Read the model definition and answer for the solid it produces. Units are mm, in the model's axes. Face numbers are marked on the shaded views. A direction names the side the tool comes from. Round coordinates to 2 decimals unless told otherwise and drop trailing zeros. Loops run counter-clockwise (first coordinate to the right, second up) from the corner with the lowest first, then second, coordinate; pieces in that order, holes last. Notation, with made-up numbers: (46.5, -13) - (59.5, -13) arc R17 ccw to (59.5, 9) - close; hole circle Ø5 at (55, 53). An arc over 180 degrees is marked (long way). Answer as CSV lines item,"result".
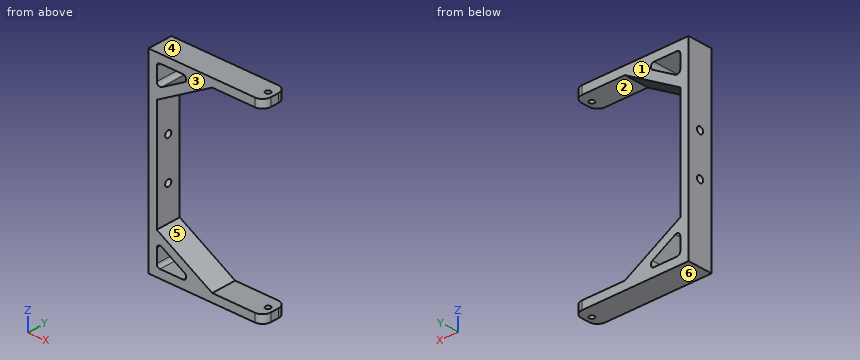
```python
from build123d import *

# Parameters (mm, degrees)
BOSS_EXTRUDE1_DEPTH     = 15
SKETCH2_R               = 1.55
CUT_EXTRUDE1_DEPTH      = 1
CUT_EXTRUDE1_DEPTH_BACK = 116
FILLET1_R               = 2
FILLET2_R               = 5
SKETCH3_R               = 2
CUT_EXTRUDE2_DEPTH      = 6


with BuildPart() as part:
    # Sketch1 → Boss-Extrude1 (new body)
    with BuildSketch(Plane(origin=(0, 0, 0), x_dir=(1, 0, 0), z_dir=(0, 1, 0))):
        Polygon((61.707917854, 52.5), (66.707917854, 52.5), (66.707917854, 57.5), (62.241203502, 57.5), (34.92783027, 57.5), (-2.5, 57.5), (-2.5, 36.198924731), (-2.5, 33.198924731), (-2.5, -33.198924731), (-2.5, -36.198924731), (-2.5, -57.5), (34.92783027, -57.5), (62.241203502, -57.5), (66.707917854, -57.5), (66.707917854, -52.5), (61.707917854, -52.5), (35.930443006, -52.5), (2.5, -33.198924731), (2.5, 33.198924731), (35.930443006, 52.5), align=None)
        Polygon((2.5, 39.085676077), (25.734290584, 52.5), (2.5, 52.5), align=None, mode=Mode.SUBTRACT)
        Polygon((2.5, -52.5), (2.5, -39.085676077), (25.734290584, -52.5), align=None, mode=Mode.SUBTRACT)
    extrude(amount=BOSS_EXTRUDE1_DEPTH)

    # Sketch2 → Cut-Extrude1 (cut, two sides)
    with BuildSketch(Plane.XY.offset(57.5)) as cut_extrude1_sk:
        with Locations((62.707917854, 7.5)):
            Circle(SKETCH2_R)
    extrude(amount=CUT_EXTRUDE1_DEPTH, mode=Mode.SUBTRACT)
    extrude(cut_extrude1_sk.sketch, amount=-CUT_EXTRUDE1_DEPTH_BACK, mode=Mode.SUBTRACT)

    # Fillet1
    fillet1_edges = [part.edges().sort_by_distance(p)[0] for p in [
        (25.734290584, 7.5, -52.5),
        (2.5, 7.5, -52.5),
        (2.5, 7.5, -39.085676077),
        (2.5, 7.5, 52.5),
        (25.734290584, 7.5, 52.5),
        (2.5, 7.5, 39.085676077),
    ]]
    fillet(fillet1_edges, radius=FILLET1_R)

    # Fillet2
    fillet2_edges = [part.edges().sort_by_distance(p)[0] for p in [
        (66.707917854, 15, -55),
        (66.707917854, 0, 55),
        (66.707917854, 0, -55),
        (66.707917854, 15, 55),
    ]]
    fillet(fillet2_edges, radius=FILLET2_R)

    # Sketch3 → Cut-Extrude2 (cut, through all)
    with BuildSketch(Plane(origin=(2.5, 0, 0), x_dir=(0, 0, -1), z_dir=(1, 0, 0))):
        with Locations((-12.5, 7.5)):
            Circle(SKETCH3_R)
        with Locations((12.5, 7.5)):
            Circle(SKETCH3_R)
    extrude(amount=-CUT_EXTRUDE2_DEPTH, mode=Mode.SUBTRACT)


solid = part.part
```
1) A cutting plane is placed at C-C, the plane x = 8.5. Determine the outline of the cut face in (y, z), plus the area to 3 significant figures.
Entries:
outline,"(0, -57.5) - (15, -57.5) - (15, -52.5) - (0, -52.5) - close; (0, -42.55) - (15, -42.55) - (15, -36.66) - (0, -36.66) - close; (0, 36.66) - (15, 36.66) - (15, 42.55) - (0, 42.55) - close; (0, 52.5) - (15, 52.5) - (15, 57.5) - (0, 57.5) - close"
area,"327 mm^2"
2) A cutting plane is placed at B-B, the plane z = -12.5. Determine the outline of the cut face in (x, y).
Entries:
outline,"(-2.5, 0) - (2.5, 0) - (2.5, 5.5) - (-2.5, 5.5) - close; (-2.5, 9.5) - (2.5, 9.5) - (2.5, 15) - (-2.5, 15) - close"
3) A cutting plane is placed at D-D, the plane y = 7.5. Count the separate pieces of the cut face and the enclosed holes in it, plus the area to 3 significant figures.
Entries:
separate pieces,"5"
enclosed holes,"2"
area,"1,510 mm^2"
4) A cutting plane is placed at A-A, the plane x = 53.5. Determine the outline of the cut face in (y, z), plus the area to 3 significant figures.
Entries:
outline,"(0, -57.5) - (15, -57.5) - (15, -52.5) - (0, -52.5) - close; (0, 52.5) - (15, 52.5) - (15, 57.5) - (0, 57.5) - close"
area,"150 mm^2"
5) The mould has two halves that part along Z. Classify the marked faces 3, 4, 5 and 6: pulls with the +Z half, pulls with the -Z half, needs draft (parallel to the pull), parting line crosses it, or undercut.
Entries:
face 3,"needs draft"
face 4,"pulls with the +Z half"
face 5,"undercut"
face 6,"pulls with the -Z half"
6) Find the intervals of material crossed by line 1 (Z direction, x = 59, y = 8); line 2 (Z direction, x = 15, y = 10.25); line 3 (Z direction, x = 20, y = 9.75), in increasing order.
Entries:
line 1,"z = -57.5 to -52.5, 52.5 to 57.5"
line 2,"z = -57.5 to -52.5, -46.3 to -40.42, 40.42 to 46.3, 52.5 to 57.5"
line 3,"z = -57.5 to -51.5, -49.5 to -43.3, 43.3 to 49.5, 51.5 to 57.5"
7) Each of these flat-tipped pins is pushed along its axis until it touches: P1, Ø5, axis at y = 7.5, z = 12.5, coming from the +X side; P2, Ø3.5, axis at x = 62.71, y = 7.5, coming from the +Z side; P3, Ø2.5, axis at y = 10.5, z = 47, coming from the +X side; P4, Ø12, axis at x = 24.5, z = -34.5, coming from the +Y side. Where does it stop, or does it pass through?
Entries:
P1,"stops at x = 2.5"
P2,"stops at z = 57.5"
P3,"stops at x = 28.57"
P4,"passes through"
8) A tool of negligible diameter and unlimited length cuts with its end or side. For the marked faces 1 and 2, from which of +Z, -Z, +X, -X, +Y, -Y can it reach the whole face along a straight path? Write none if from no direction.
Entries:
face 1,"+Z, -Z, +X, -X, +Y"
face 2,"+X, +Y, -Y"
